Autodesk Inventor part; units mm, degrees
ref_plane "YZ Plane" through (0, 0, 0) normal (1, 0, 0) x (0, 1, 0)
ref_plane "XZ Plane" through (0, 0, 0) normal (0, 1, 0) x (-1, 0, 0)
ref_plane "XY Plane" through (0, 0, 0) normal (0, 0, 1) x (1, 0, 0)
sketch "Sketch6" plane through (0, 0, 0) normal (0, 0, 1) x (1, 0, 0)
  circle A0 centre (0, 0) radius 2.75
  line L0 (0, 0) -> (0, 125)
  line L1 (0, 0) -> (108.2532, 62.5)
  line L2 (0, 0) -> (125, 0) construction
  line L3 (0, 0) -> (18.8687, 32.6815)
  line L4 (0, 0) -> (37.7374, 0) construction
  line L5 (108.2532, 62.5) -> (9.497, 16.4492)
  line L6 (108.2532, 62.5) -> (217.2186, 62.5) construction
  line L7 (9.497, 16.4492) -> (0, 125)
  line L8 (0, 125) -> (-9.497, 16.4492)
  line L9 (-9.497, 16.4492) -> (-108.2532, 62.5)
  line L10 (-108.2532, 62.5) -> (-18.9939, 0)
  line L11 (-18.9939, 0) -> (-108.2532, -62.5)
  line L12 (-108.2532, -62.5) -> (-9.497, -16.4492)
  line L13 (-9.497, -16.4492) -> (0, -125)
  line L14 (0, -125) -> (9.497, -16.4492)
  line L15 (9.497, -16.4492) -> (108.2532, -62.5)
  line L16 (108.2532, -62.5) -> (18.9939, 0)
  line L17 (18.9939, 0) -> (108.2532, 62.5)
  dimension "d21" = 5.5
  dimension "d22" = 125
  dimension "d23" = 30
  dimension "d24" = 60
  dimension "d25" = 155
  dimension "d28" = 360
extrude "Extrusion2" add sketch "Sketch6" along normal blind 76.2 contours L1 L3 A0 | A0 L3 L5 L1 | L0 L7 L3 A0 | A0 L3 L0
sketch "Sketch4" plane through (0, 0, 0) normal (0, 1, 0) x (-1, 0, 0)
  line L0 (-125.0691, 0) -> (-125.0691, 76.2)
  line L1 (0, -15.24) -> (0, 91.44)
  line L2 (-50.0691, 0) -> (-0.0691, 0)
  line L3 (-50, 76.2) -> (0, 76.2)
  line L4 (0, 76.2) -> (-125.0691, 76.2)
  line L5 (0, 0) -> (-108.2532, 0)
  line L6 (-125.0691, 0) -> (0, 0)
  arc A0 (-50, 76.2) -> (-50.0691, 0) centre (1.6634, 38.0531) ccw
  point P0 (-25, 76.2)
  point P1 (-0.0691, 76.2)
  point P2 (-62.5691, 76.2)
  dimension "d7" = 125
  dimension "d36" = 50
  dimension "d37" = 50
pattern_circular "Circular Pattern1" count 6 over 360 about axis through (0, 0, -10) along (0, 0, 1) of "Extrusion2"
revolve "Revolution2" cut sketch "Sketch4" angle 360 about axis through (0, 0, -10) along (0, 0, 1) contours L0 L4 A0 L5 L6
fillet "Fillet1" radius 5 1 edges at (-18.9939, 0, 38.1)
pattern_circular "Circular Pattern2" count 6 over 360 about axis through (0, 0, -10) along (0, 0, 1) of "Fillet1"
sketch "Sketch9" plane through (0, 0, 76.2) normal (0, 0, 1) x (1, 0, 0)
  circle A0 centre (0, 0) radius 2.5
  line L0 (0, 2.5) -> (0, 2.02)
  line L1 (0, 2.02) -> (-1.473, 2.02)
  line L2 (0, 2.02) -> (1.473, 2.02)
  dimension "d42" = 5
  dimension "d43" = 0.48
extrude "Extrusion3" cut sketch "Sketch9" against normal blind 14 contours A0 L1 L2
sketch "Sketch10" plane through (0, 0, 76.2) normal (0, 0, 1) x (1, 0, 0)
  point P0 (0, 0)
properties part number "Dispensing Gear V2"
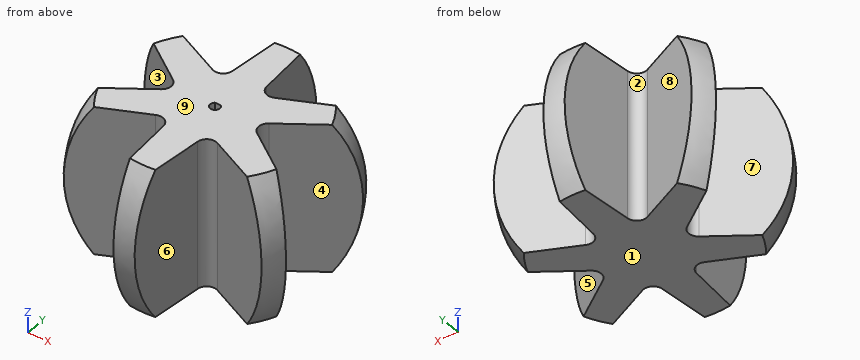
Geometry: final body of the model. Coordinates: model frame, mm. Face numbers are marked on the shaded views. A direction names the side the tool comes from. Coordinates: 2 decimals unless noted, no trailing zeros. Loops run counter-clockwise (first coordinate to the right, second up) from the corner with the lowest first, then second, coordinate; pieces in that order, holes last. Notation, with made-up numbers: (82, 24.5) - (123, 24.5) arc R19 cw to (123, 32.5) - close; hole circle Ø11 at (-11, 37). An arc over 180 degrees is marked (long way). One line per question, with ' | ' between items. Start each with the question number.
(1) First-contact query: pin 1 (2.5 mm diameter, centred on x = 0.5, y = 0.5, fed in from +Z); pin 2 (12 mm diameter, centred on y = 50, z = 57.5, fed in from +X); pin 3 (12 mm diameter, centred on x = -19, z = 60, fed in from +Y); pin 4 (6 mm diameter, centred on x = 0, y = 0, fed in from +Z). Flat tips, straight axial feed; report the tip coordinate or a pass-through.
(2) Cut plane C-C on y = 47.5. Output: boundary loops of the cut face in (x, z).
(3) Ray query, L1, parallel to X at y = -27.5, z = 21; L2, parallel to X at y = 35, z = 24.5; L3, parallel to X at y = 0, z = 69.5. Return the intervals inside material, ascending. Write a range as from..to.
(4) Reachability of the marked faces 5, 6, 7, 8 and 9 from +Z, -Z, +X, -X, +Y, -Y: full face, straight path, thin tool, end or side. Return the list, or none.
(5) Cut plane A-A on y = 0. Output: boundary loops of the cut face in (x, z).
(6) Cut plane B-B on x = -18. Output: boundary loops of the cut face in (y, z).
(7) Draft query along X for the marked faces 1, 2, 3 and 4. Return one class per face: +X half, -X half, draft (parallel to the pull), parting line (faces both ways), or undercut.
Here are the results:
1) pin 1: z = 62.2 | pin 2: x = 7.09 | pin 3: y = 23.68 | pin 4: z = 76.2
2) outline: (-6.78, 0) - (6.78, 0) - (6.78, 76.2) - (-6.78, 76.2) - close
3) L1: -53.61..-33.2, -8.53..8.53, 33.2..53.61 | L2: -50.1..-49.28, -7.87..7.87, 49.28..50.1 | L3: -22.71..-2.5, 2.5..22.71
4) face 5: +Z, -Z, +X | face 6: +Z, -Z, -Y | face 7: +Z, -Z, -X | face 8: +Z, -Z, +Y | face 9: +Z, +X, -X, +Y, -Y
5) outline: (-22.71, 0) - (22.71, 0) - (22.71, 76.2) - (2.5, 76.2) - (2.5, 62.2) - (-2.5, 62.2) - (-2.5, 76.2) - (-22.71, 76.2) - close
6) outline: (-20.41, 0) - (20.41, 0) - (20.41, 76.2) - (-20.41, 76.2) - close
7) face 1: draft | face 2: undercut | face 3: -X half | face 4: +X half
